The listing builds one solid part. Answer for the finished solid, in the listing's coordinates (mm). Face numbers are marked on the shaded views. A direction names the side the tool comes from. Coordinates: 2 decimals unless noted, no trailing zeros. Write each loop counter-clockwise with the first axis right and the second up, starting at its lowest first coordinate (ties: lowest second). Pieces come first, ordered by that corner, then holes.
(1) The part is cut by section A-A on y = 68. Determine the outline of the cut face in (x, z).
(2) Which of the six approach directions +Z, -Z, +X, -X, +Y, -Y give full straight-line access (tool end or side, diameter ignored) to the marked faces 1 and 2?
(3) Given P1, Ø10, axis at x = 38, y = -42.5, coming from the -Z side, flat-ended and moving along its own axis, determine where the tip first touches the part or whether it passes through.
(4) Straight lines are drawn through the part: line 1 (Y direction, x = 2.5, z = 39); line 2 (X direction, y = -24, z = 23); line 3 (Z direction, x = -33, y = -4). For each, find the intervals that lie inside material, in ascending order.
(5) The part is cut by section B-B on z = 15. Determine the outline of the cut face in (x, y).
(6) For a pull along Y with two mould halves and no side action, classify the marked faces 3, 4, 5 and 6 as +Y half, -Y half, draft (parallel to the pull), parting line (faces both ways), or undercut.
(7) The part is cut by section C-C on x = 14. Determine the outline of the cut face in (y, z).
from build123d import *

# Parameters (mm, degrees)
F0_W     = 203.2
F0_H     = 203.2
F0_W_2   = 76.2
F0_H_2   = 165.1
F1_DEPTH = 5.08
F2_DEPTH = 50.8
F3_SIZE  = 5.08


with BuildPart() as f1:
    # F0 (on Top) → F1 (new body)
    with BuildSketch(Plane.XY):
        Rectangle(F0_W, F0_H)
        Rectangle(F0_W_2, F0_H_2, mode=Mode.SUBTRACT)
        Rectangle(F0_W_2, F0_H_2)
    extrude(amount=F1_DEPTH)

    # F0 (on Top) → F2 (join)
    with BuildSketch(Plane.XY):
        Rectangle(F0_W, F0_H)
        Rectangle(F0_W_2, F0_H_2, mode=Mode.SUBTRACT)
    extrude(amount=F2_DEPTH)

    # F3
    f3_edges = [f1.edges().sort_by_distance(p)[0] for p in [
        (-38.1, 0, 50.8),
        (38.1, 0, 50.8),
    ]]
    chamfer(f3_edges, length=F3_SIZE)


solid = f1.part
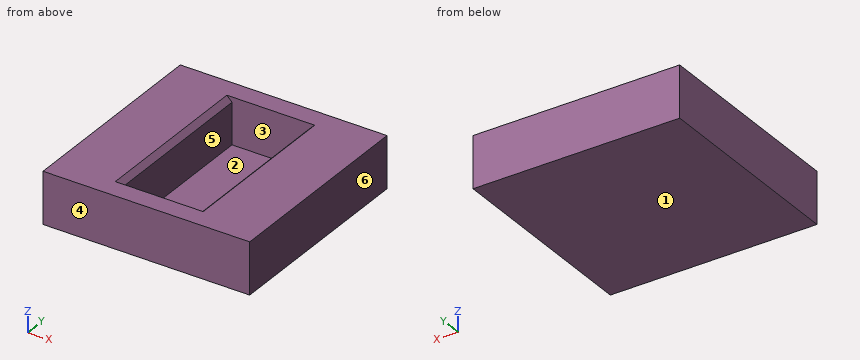
Model answer:
1. outline: (-101.6, 0) - (101.6, 0) - (101.6, 50.8) - (43.18, 50.8) - (38.1, 45.72) - (38.1, 5.08) - (-38.1, 5.08) - (-38.1, 45.72) - (-43.18, 50.8) - (-101.6, 50.8) - close
2. face 1: -Z, +X, -X, +Y, -Y
2. face 2: +Z
3. P1: stops at z = 0
4. line 1: y = -101.6 to -82.55, 82.55 to 101.6
4. line 2: x = -101.6 to -38.1, 38.1 to 101.6
4. line 3: z = 0 to 5.08
5. outline: (-101.6, -101.6) - (101.6, -101.6) - (101.6, 101.6) - (-101.6, 101.6) - close; hole (-38.1, -82.55) - (38.1, -82.55) - (38.1, 82.55) - (-38.1, 82.55) - close
6. face 3: undercut
6. face 4: -Y half
6. face 5: undercut
6. face 6: draft
7. outline: (-101.6, 0) - (101.6, 0) - (101.6, 50.8) - (82.55, 50.8) - (82.55, 5.08) - (-82.55, 5.08) - (-82.55, 50.8) - (-101.6, 50.8) - close
